```python
from build123d import *

# Parameters (mm, degrees)
SKETCH_1_W          = 68
SKETCH_1_H          = 27
EXTRUDE_1_DEPTH     = 7
SKETCH_2_W          = 63.5
SKETCH_2_H          = 22.5
CUT_EXTRUDE_1_DEPTH = 4.5
EXTRUDE_2_DEPTH     = 2.9
EXTRUDE_3_DEPTH     = 4.5
SKETCH_5_R          = 1.2
CUT_EXTRUDE_2_DEPTH = 37.978507271
CUT_EXTRUDE_3_DEPTH = 2
SKETCH_7_W          = 10
SKETCH_7_H          = 19
CUT_EXTRUDE_4_DEPTH = 5
FILLET_1_R          = 2
FILLET_2_R          = 1


with BuildPart() as part:
    # Эскиз1 → Бобышка-Вытянуть1 (new body)
    with BuildSketch(Plane(origin=(0, 0, 0), x_dir=(1, 0, 0), z_dir=(0, 1, 0))):
        Rectangle(SKETCH_1_W, SKETCH_1_H)
    extrude(amount=EXTRUDE_1_DEPTH)

    # Эскиз2 → Вырез-Вытянуть1 (cut)
    with BuildSketch(Plane(origin=(0, 7, 0), x_dir=(1, 0, 0), z_dir=(0, 1, 0))):
        Rectangle(SKETCH_2_W, SKETCH_2_H)
    extrude(amount=-CUT_EXTRUDE_1_DEPTH, mode=Mode.SUBTRACT)

    # Эскиз3 → Бобышка-Вытянуть2 (add)
    with BuildSketch(Plane(origin=(0, 2.5, 0), x_dir=(1, 0, 0), z_dir=(0, 1, 0))):
        with BuildLine():
            Line((-23.5, 9), (-23.5, 11.25))
            Line((-23.5, 11.25), (-19.5, 11.25))
            Line((-19.5, 11.25), (-19.5, 9))
            ThreePointArc((-19.5, 9), (-21.5, 7), (-23.5, 9))
        make_face()
        with BuildLine():
            Line((-19.5, -11.25), (-19.5, -9))
            ThreePointArc((-19.5, -9), (-21.5, -7), (-23.5, -9))
            Line((-23.5, -9), (-23.5, -11.25))
            Line((-23.5, -11.25), (-19.5, -11.25))
        make_face()
    extrude(amount=EXTRUDE_2_DEPTH)

    # Эскиз4 → Бобышка-Вытянуть3 (add)
    with BuildSketch(Plane(origin=(0, 2.5, 0), x_dir=(1, 0, 0), z_dir=(0, 1, 0))):
        with BuildLine():
            Line((22.3, 11), (22.3, 11.25))
            Line((22.3, 11.25), (23.7, 11.25))
            Line((23.7, 11.25), (23.7, 11))
            ThreePointArc((23.7, 11), (23, 10.3), (22.3, 11))
        make_face()
        with BuildLine():
            Line((23.7, -11.25), (23.7, -11))
            ThreePointArc((23.7, -11), (23, -10.3), (22.3, -11))
            Line((22.3, -11), (22.3, -11.25))
            Line((22.3, -11.25), (23.7, -11.25))
        make_face()
    extrude(amount=EXTRUDE_3_DEPTH)

    # Эскиз5 → Вырез-Вытянуть2 (cut, through all)
    with BuildSketch(Plane(origin=(0, 5.4, 0), x_dir=(1, 0, 0), z_dir=(0, 1, 0))):
        with Locations(Location((-21.5, 9, 0), (0, 0, 270))):
            Circle(SKETCH_5_R)
        with Locations(Location((-21.5, -9, 0), (0, 0, 270))):
            Circle(SKETCH_5_R)
    extrude(amount=-CUT_EXTRUDE_2_DEPTH, mode=Mode.SUBTRACT)

    # Эскиз6 → Вырез-Вытянуть3 (cut)
    with BuildSketch(Plane.XZ):
        with BuildLine():
            Line((-19.5, -9), (-19.5, -13.5))
            Line((-19.5, -13.5), (-23.5, -13.5))
            Line((-23.5, -13.5), (-23.5, -9))
            ThreePointArc((-23.5, -9), (-21.5, -7), (-19.5, -9))
        make_face()
        with BuildLine():
            Line((-23.5, 13.5), (-23.5, 9))
            ThreePointArc((-23.5, 9), (-21.5, 7), (-19.5, 9))
            Line((-19.5, 9), (-19.5, 13.5))
            Line((-19.5, 13.5), (-23.5, 13.5))
        make_face()
    extrude(amount=-CUT_EXTRUDE_3_DEPTH, mode=Mode.SUBTRACT)

    # Эскиз7 → Вырез-Вытянуть4 (cut)
    with BuildSketch(Plane.XZ):
        with Locations((29, 0)):
            Rectangle(SKETCH_7_W, SKETCH_7_H)
    extrude(amount=-CUT_EXTRUDE_4_DEPTH, mode=Mode.SUBTRACT)

    # Скругление1
    fillet_1_edges = [part.edges().sort_by_distance(p)[0] for p in [
        (-28.75, 0, -13.5),
        (7.25, 0, -13.5),
        (34, 3.5, -13.5),
        (-34, 3.5, -13.5),
        (-28.75, 0, 13.5),
        (7.25, 0, 13.5),
        (34, 0, 11.5),
        (-34, 0, 0),
        (34, 3.5, 13.5),
        (-34, 3.5, 13.5),
    ]]
    fillet(fillet_1_edges, radius=FILLET_1_R)

    # Скругление2
    fillet_2_edges = [part.edges().sort_by_distance(p)[0] for p in [
        (24, 1.25, -9.5),
        (24, 1.25, 9.5),
    ]]
    fillet(fillet_2_edges, radius=FILLET_2_R)


solid = part.part
```
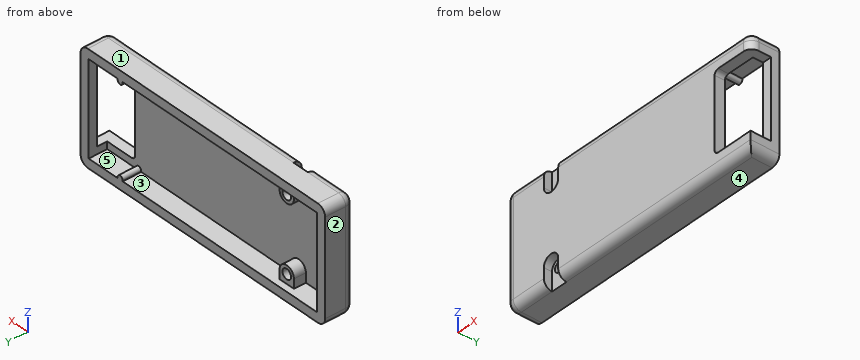
Part model, mm, in its own coordinate system. Face numbers are marked on the shaded views. A direction names the side the tool comes from. Give positions to 0.01 mm unless a question says otherwise; leave off trailing zeros. Order: outer loops, then holes, each group sorted by start corner. A loop starts at its lowest first (then second) coordinate and runs counter-clockwise, first axis right, second up. Notation, with made-up numbers: M 62,86 L 120,86 A7 ccw 120,91 Z; hole C 72,74 d8. An arc over 180 degrees is marked long. Use a Markdown table: item, result. Add a question column.
(1) Drop flat-ended pins along their axis: P1, Ø2, axis at x = -10.5, z = 9, coming from the +Y side; P2, Ø3, axis at y = 1, z = 1.5, coming from the +X side; P3, Ø1.2, axis at x = -21.5, z = 8, coming from the +Y side; P4, Ø2, axis at x = -21.5, z = 9, coming from the -Y side. Give the stop position or say it passes through.
(2) Saw through at C-C, the plane y = 3.5. Give the number of separate pieces and of enclosed holes in the cut face, and give its area (3 significant figures).
(3) Saw through at D-D, the plane x = 1. Give the cut face in (y, z).
(4) 3-axis set-ups, long thin cutter, end or side, ignore diameter. For the marked faces 4 and 5: which of +Z, -Z, +X, -X, +Y, -Y reach the whole face in a straight line?
(5) Mould opens along X. For the marked faces 1, 2 and 3 say: +X half, -X half, draft (parallel to the pull), parting line (faces both ways), or undercut.
(6) Probe line 1 along X through (y, z) = (3, 9); line 2 along X through (y, z) = (6.25, -7.25); line 3 along Z through (x, y) = (11, 3). List the from-to ranges inside material, lowest first. Write a range as [from, to].
(7) Saw through at B-B, the plane z = 1.5. Give the cut face in (x, y), and give its area (3 significant figures).
(8) Saw through at A-A, the plane x = -21.5. Give the cut face in (y, z), and give its area (3 significant figures).
Answer key:
| question | item | result |
|---|---|---|
| 1 | P1 | y = 2.5 |
| 1 | P2 | x = 24 |
| 1 | P3 | y = 5.4 |
| 1 | P4 | through |
| 2 | separate pieces | 1 |
| 2 | enclosed holes | 2 |
| 2 | area | 385 mm^2 |
| 3 | outline | M 0,-11.5 A2 ccw 2,-13.5 L 7,-13.5 L 7,-11.25 L 2.5,-11.25 L 2.5,11.25 L 7,11.25 L 7,13.5 L 2,13.5 A2 ccw 0,11.5 Z |
| 4 | face 4 | -Z, +X, -X, +Y, -Y |
| 4 | face 5 | +Y |
| 5 | face 1 | draft |
| 5 | face 2 | -X half |
| 5 | face 3 | undercut |
| 6 | line 1 | [-34, -31.75], [-23.5, -22.7], [-20.3, -19.5] |
| 6 | line 2 | [-34, -31.75], [31.75, 34] |
| 6 | line 3 | [-13.5, -11.25], [11.25, 13.5] |
| 7 | outline | M -34,2 A2 ccw -32,0 L 24,0 L 24,2.5 L -31.75,2.5 L -31.75,7 L -34,7 Z; M 31.75,5 L 34,5 L 34,7 L 31.75,7 Z |
| 7 | area | 159 mm^2 |
| 8 | outline | M 0,-7 L 2,-7 L 2,-7.8 L 5.4,-7.8 L 5.4,-7 L 2.5,-7 L 2.5,7 L 5.4,7 L 5.4,7.8 L 2,7.8 L 2,7 L 0,7 Z; M 2,-13.5 L 7,-13.5 L 7,-11.25 L 5.4,-11.25 L 5.4,-10.2 L 2,-10.2 Z; M 2,10.2 L 5.4,10.2 L 5.4,11.25 L 7,11.25 L 7,13.5 L 2,13.5 Z |
| 8 | area | 70.1 mm^2 |
